Work out the finished part from the listing and answer in its coordinate system (mm). A direction names the side the tool comes from. Coordinates: 2 decimals unless noted, no trailing zeros. Order: outer loops, then holes, each group sorted by start corner. A loop starts at its lowest first (then second) coordinate and runs counter-clockwise, first axis right, second up. Notation, with made-up numbers: M -15,43.5 L 42,43.5 A7 cw 42,53.5 Z; hole C 79.25,86.5 d2. An arc over 180 degrees is marked long. Use a Markdown table: item, result.
from build123d import *

# Parameters (mm, degrees)
SKETCH1_R           = 5
BOSS_EXTRUDE1_DEPTH = 70
SKETCH3_R           = 3.5
BOSS_EXTRUDE2_DEPTH = 7
SKETCH4_R           = 2.5
BOSS_EXTRUDE3_DEPTH = 7
SKETCH7_OUTSIDE_W   = 29.036
SKETCH7_OUTSIDE_H   = 29.036
SKETCH7_OUTSIDE_R   = 2
CUT_EXTRUDE5_DEPTH  = 2
CHAMFER1_SIZE       = 0.5
FILLET1_R           = 0.5
SKETCH8_R           = 9
BOSS_EXTRUDE4_DEPTH = 15


with BuildPart() as part:
    # Sketch1 → Boss-Extrude1 (new body)
    with BuildSketch(Plane(origin=(0, 0, 0), x_dir=(0, 0, -1), z_dir=(1, 0, 0))):
        Circle(SKETCH1_R)
    extrude(amount=BOSS_EXTRUDE1_DEPTH)

    # Sketch3 → Boss-Extrude2 (add)
    with BuildSketch(Plane.ZY):
        Circle(SKETCH3_R)
    extrude(amount=BOSS_EXTRUDE2_DEPTH)

    # Sketch4 → Boss-Extrude3 (add)
    with BuildSketch(Plane.ZY.offset(7)):
        Circle(SKETCH4_R)
    extrude(amount=BOSS_EXTRUDE3_DEPTH)

    # Sketch7 outside → Cut-Extrude5 (cut)
    with BuildSketch(Plane.ZY.offset(7)):
        Rectangle(SKETCH7_OUTSIDE_W, SKETCH7_OUTSIDE_H)
        Circle(SKETCH7_OUTSIDE_R, mode=Mode.SUBTRACT)
    extrude(amount=CUT_EXTRUDE5_DEPTH, mode=Mode.SUBTRACT)

    # Chamfer1
    chamfer1_edges = [part.edges().sort_by_distance(p)[0] for p in [
        (-14, 0, -2.5),
    ]]
    chamfer(chamfer1_edges, length=CHAMFER1_SIZE)

    # Fillet1
    fillet1_edges = [part.edges().sort_by_distance(p)[0] for p in [
        (-7, 0, -2),
        (-9, 0, -2),
    ]]
    fillet(fillet1_edges, radius=FILLET1_R - 0.0001)  # a hair under: the kernel refuses the full size

    # Sketch8 → Boss-Extrude4 (add)
    with BuildSketch(Plane(origin=(70, 0, 0), x_dir=(0, 0, -1), z_dir=(1, 0, 0))):
        Circle(SKETCH8_R)
    extrude(amount=BOSS_EXTRUDE4_DEPTH)


solid = part.part
1. For a pull along X with two mould halves and no side action, classify faces 3 (the face through (-7, -2, 2)), 4 (the face through (-8, -2, 0)), 5 (the face through (-3.451, -1.341, 3.233)) as +X half, -X half, draft (parallel to the pull), parting line (faces both ways), or undercut.
Answers below:
| item | result |
|---|---|
| face 3 | -X half |
| face 4 | undercut |
| face 5 | draft |
2. Section C-C on x = 24 is taken. Determine the outline of the cut face in (y, z).
Answers below:
| item | result |
|---|---|
| outline | C 0,0 d10 |
3. Flat-ended cylindrical pins translate along their axes: P1, Ø5, axis at x = 54.5, y = 2.5, coming from the +Z side; P2, Ø2, axis at x = 61, y = 2.5, coming from the +Z side; P3, Ø3, axis at x = 1, z = 4, coming from the +Y side; P4, Ø3, axis at y = 0.5, z = -2, coming from the -X side. Find the tip coordinate at first contact, or state that the pin passes through.
Answers below:
| item | result |
|---|---|
| P1 | z = 5 |
| P2 | z = 4.77 |
| P3 | y = 4.33 |
| P4 | x = -14 |
4. For faces 1 (the face through (-11.22, -2.44, -0.54)), 2 (the face through (-14, 0, 0)), determine the directions among +Z, -Z, +X, -X, +Y, -Y from which every point of the face is accessible in a straight line to the end or side of a thin tool.
Answers below:
| item | result |
|---|---|
| face 1 | -X |
| face 2 | +Z, -Z, -X, +Y, -Y |
5. Find the intervals of material crossed by probe 1 along X at (y, z) = (-1.5, 1.75); probe 2 along X at (y, z) = (-1, -3.25); probe 3 along X at (y, z) = (5, -2.25), in increasing order.
Answers below:
| item | result |
|---|---|
| probe 1 | -13.7 to -8.96, -7.04 to 85 |
| probe 2 | -7 to 85 |
| probe 3 | 70 to 85 |
6. Section D-D on x = -3 is taken. Determine the outline of the cut face in (y, z), then the cut area to 3 significant figures.
Answers below:
| item | result |
|---|---|
| outline | C 0,0 d7 |
| area | 38.5 mm² |
